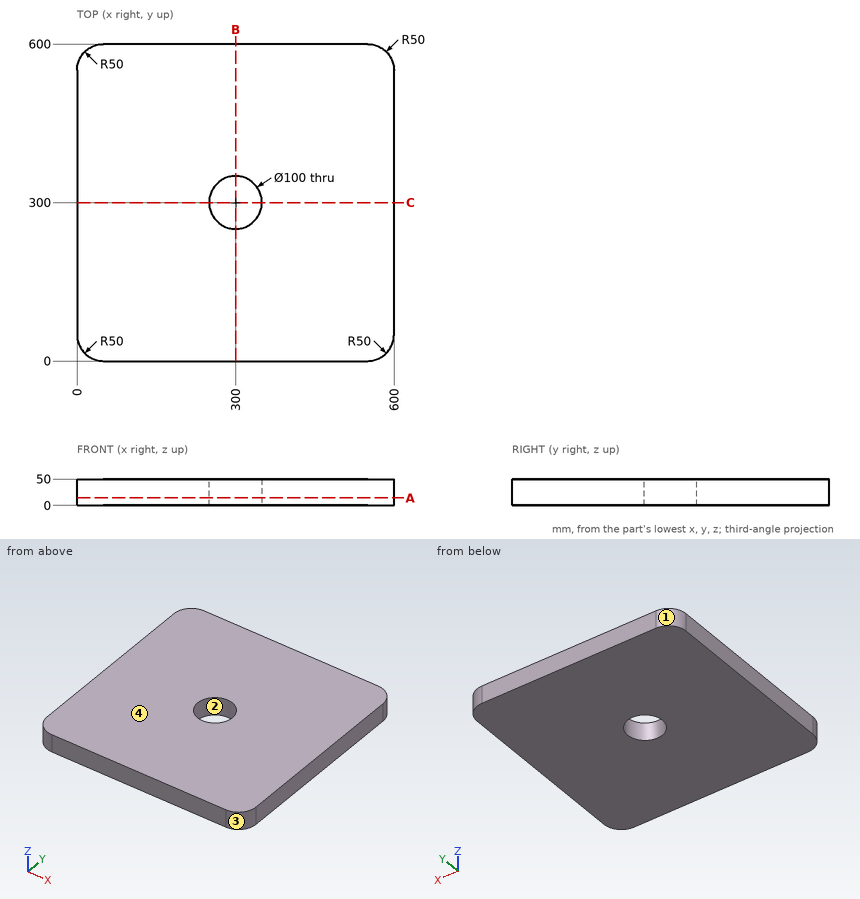
Geometry: see drawing. Coordinates: mm, zero at the bounding-box minimum. Give positions to 0.01 mm unless a question says otherwise; leave off trailing zeros. Write each loop counter-clockwise with the first axis right and the second up, starting at its lowest first coordinate (ties: lowest second). Pieces come first, ordered by that corner, then holes. Notation, with made-up numbers: (33.25, -1) - (44.25, -1) arc R14 cw to (44.25, 9) - close; hole circle Ø3 at (-4, 62.5). An arc over 180 degrees is marked (long way). Return JSON: item names as keys, results as strings. Group by question number.
1) Section B-B on x = 300. Return the cut outline in (y, z), plus the area to 3 significant figures.
2) Line query: line 1 (Y direction, x = 300, z = 24.5); line 2 (Y direction, x = 260.5, z = 17); line 3 (X direction, y = 267, z = 4). Output: solid intervals per line, ascending.
3) Mould query, pull axis Y, two halves, no side actions, for the marked faces 1, 2, 3 and 4. Classes: released by +Y, released by -Y, zero draft, split by the parting line, or undercut.
4) Section A-A on z = 14.5. Return the cut outline in (x, y).
Filled in:
{
 "1": {"outline": "(0, 0) - (250, 0) - (250, 50) - (0, 50) - close; (350, 0) - (600, 0) - (600, 50) - (350, 50) - close", "area": "25,000 mm^2"},
 "2": {"line 1": "y = 0 to 250, 350 to 600", "line 2": "y = 0 to 269.34, 330.66 to 600", "line 3": "x = 0 to 262.44, 337.56 to 600"},
 "3": {"face 1": "released by +Y", "face 2": "undercut", "face 3": "released by -Y", "face 4": "zero draft"},
 "4": {"outline": "(0, 50) arc R50 ccw to (50, 0) - (550, 0) arc R50 ccw to (600, 50) - (600, 550) arc R50 ccw to (550, 600) - (50, 600) arc R50 ccw to (0, 550) - close; hole circle Ø100 at (300, 300)"}
}
